Study the drawing (mm; zero at the part's minimum x, y, z) and answer. A direction names the side the tool comes from. Give positions to 0.01 mm unless a question says otherwise; leave off trailing zeros. Write each loop counter-clockwise with the first axis right and the second up, starting at its lowest first coordinate (ties: lowest second). Pieces come first, ordered by that corner, then holes.
1) Given pin 1 Ø1.5 at (x, y) = (12.5, 4) entering from -Z; pin 2 Ø2 at (x, z) = (37.5, 12) entering from +Y; pin 3 Ø1.5 at (x, y) = (7, 2.5) entering from -Z, each flat-ended and moving along its own axis, determine where each tip first touches the part or whether it passes through.
2) Find section D-D (y = 2). Determine the outline of the cut face in (x, z).
3) Determine the mould class of the marked faces 1, 2, 3 and 4 for opening direction X: pulls with the +X half, pulls with the -X half, needs draft (parallel to the pull), parting line crosses it, or undercut.
4) Find section B-B (y = 5). Determine the outline of the cut face in (x, z).
5) Straight lines are drawn through the part: probe 1 along X at (y, z) = (7.5, 15.75); probe 2 along X at (y, z) = (1, 18); probe 3 along Z at (x, y) = (5, 6.75). For each, find the intervals that lie inside material, in ascending order.
6) A tool of negligible diameter and unlimited length cuts with its end or side. For the marked faces 5, 6 and 7, from which of +Z, -Z, +X, -X, +Y, -Y can it reach the whole face along a straight path? Write none if from no direction.
7) Find section C-C (z = 18.5). Determine the outline of the cut face in (x, y).
8) Find section A-A (x = 37). Determine the outline of the cut face in (y, z), plus the area to 3 significant figures.
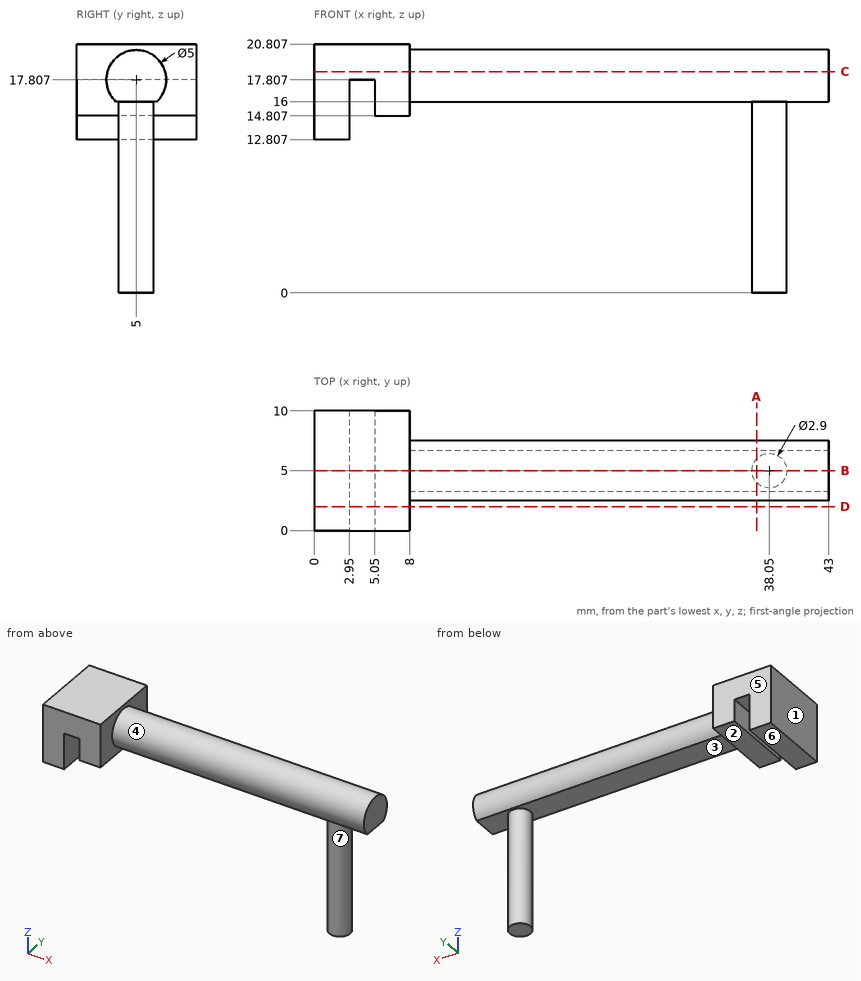
Results:
1. pin 1: stops at z = 16
1. pin 2: stops at y = 6.45
1. pin 3: stops at z = 14.81
2. outline: (0, 12.81) - (2.95, 12.81) - (2.95, 17.81) - (5.05, 17.81) - (5.05, 14.81) - (8, 14.81) - (8, 20.81) - (0, 20.81) - close
3. face 1: pulls with the -X half
3. face 2: undercut
3. face 3: undercut
3. face 4: needs draft
4. outline: (0, 12.81) - (2.95, 12.81) - (2.95, 17.81) - (5.05, 17.81) - (5.05, 14.81) - (8, 14.81) - (8, 16) - (36.6, 16) - (36.6, 0) - (39.5, 0) - (39.5, 16) - (43, 16) - (43, 20.31) - (8, 20.31) - (8, 20.81) - (0, 20.81) - close
5. probe 1: x = 0 to 2.95, 5.05 to 8
5. probe 2: x = 0 to 8
5. probe 3: z = 17.81 to 20.81
6. face 5: +Z, -Z, +X, -X, +Y
6. face 6: -Z, -X, +Y, -Y
6. face 7: -Z
7. outline: (0, 0) - (8, 0) - (8, 2.6) - (43, 2.6) - (43, 7.4) - (8, 7.4) - (8, 10) - (0, 10) - close
8. outline: (3.27, 16) - (4, 16) - (4, 0) - (6, 0) - (6, 16) - (6.73, 16) arc R2.5 ccw (long way) to start
8. area: 50.0 mm2
